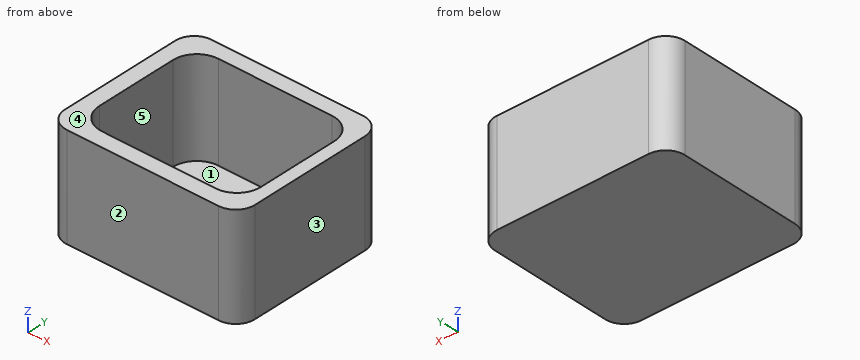
from build123d import *

# Parameters (mm, degrees)
F0_W     = 50.268072
F0_H     = 42.637728
F1_DEPTH = 27.178
F3_DEPTH = 25.4
F4_R     = 5.08
F5_R     = 5.08
F6_R     = 5.08
F7_R     = 5.08


with BuildPart() as f1:
    # F0 (on Top) → F1 (new body)
    with BuildSketch(Plane.XY):
        with Locations((-30.954471, -45.758236)):
            Rectangle(F0_W, F0_H)
    extrude(amount=F1_DEPTH)

    # F2 (on face) → F3 (cut)
    with BuildSketch(Plane.XY.offset(27.178)):
        with BuildLine():
            Line((-15.500558, -28.52626), (-45.524775, -28.52626))
            ThreePointArc((-45.524775, -28.52626), (-50.014904, -30.386132), (-51.874775, -34.87626))
            Line((-51.874775, -34.87626), (-51.874775, -56.50087))
            ThreePointArc((-51.874775, -56.50087), (-50.014904, -60.990998), (-45.524775, -62.85087))
            Line((-45.524775, -62.85087), (-15.500558, -62.85087))
            ThreePointArc((-15.500558, -62.85087), (-11.01043, -60.990998), (-9.150558, -56.50087))
            Line((-9.150558, -56.50087), (-9.150558, -34.87626))
            ThreePointArc((-9.150558, -34.87626), (-11.01043, -30.386132), (-15.500558, -28.52626))
        make_face()
    extrude(amount=-F3_DEPTH, mode=Mode.SUBTRACT)

    # F4
    f4_edges = [f1.edges().sort_by_distance(p)[0] for p in [
        (-56.088507, -67.0771, 13.589),
    ]]
    fillet(f4_edges, radius=F4_R)

    # F5
    f5_edges = [f1.edges().sort_by_distance(p)[0] for p in [
        (-5.820435, -67.0771, 13.589),
    ]]
    fillet(f5_edges, radius=F5_R)

    # F6
    f6_edges = [f1.edges().sort_by_distance(p)[0] for p in [
        (-56.088507, -24.439372, 13.589),
    ]]
    fillet(f6_edges, radius=F6_R)

    # F7
    f7_edges = [f1.edges().sort_by_distance(p)[0] for p in [
        (-5.820435, -24.439372, 13.589),
    ]]
    fillet(f7_edges, radius=F7_R)


solid = f1.part
The model under review builds one solid part; all positions refer to its coordinate system, in mm. Face numbers are marked on the shaded views. A direction names the side the tool comes from. Coordinates: 2 decimals unless noted, no trailing zeros. Loops run counter-clockwise (first coordinate to the right, second up) from the corner with the lowest first, then second, coordinate; pieces in that order, holes last. Notation, with made-up numbers: (47.25, -36.75) -> (98.25, -36.75) arc R9 ccw to (98.25, -19.75) -> close; hole circle Ø5 at (16, -21.5). An arc over 180 degrees is marked (long way). Use a Markdown table: item, result. Add a question column.
1. Add section C-C on x = -28. Write out the cut boundary in (y, z).
2. Machinability: for the marked faces 1 and 2, which of the approach directions +Z, -Z, +X, -X, +Y, -Y give a long, thin tool a straight path to every point of the face, cutting with its end or side? Answer none if there is none.
3. Add section B-B on y = -39. Write out the cut boundary in (x, z).
4. Add section A-A on z = 5.25. Write out the cut boundary in (x, y), plus the area to 3 significant figures.
5. Clearance check with flat-ended pins moving along their axes: pin 1 Ø10.5 at (x, y) = (-27.5, -46.5) entering from +Z; pin 2 Ø1.5 at (x, y) = (-23, -41) entering from -Z. State where each tip first meets the part, or that it passes through.
6. Draft analysis for pull direction X (two halves, no side actions). For the marked faces 3, 4 and 5, state which applies: pulls with the +X half, pulls with the -X half, needs draft (parallel to the pull), parting line crosses it, or undercut.
7. To check wall thickness, follow line 1 (X direction, y = -36.5, z = 23.75); line 2 (Y direction, x = -16, z = 6.5); line 3 (Z direction, x = -51, y = -54.5). State the ranges of each line that lie inside material, in increasing order.
Returned:
| question | item | result |
|---|---|---|
| 1 | outline | (-67.08, 0) -> (-24.44, 0) -> (-24.44, 27.18) -> (-28.53, 27.18) -> (-28.53, 1.78) -> (-62.85, 1.78) -> (-62.85, 27.18) -> (-67.08, 27.18) -> close |
| 2 | face 1 | +Z |
| 2 | face 2 | +Z, -Z, +X, -X, -Y |
| 3 | outline | (-56.09, 0) -> (-5.82, 0) -> (-5.82, 27.18) -> (-9.15, 27.18) -> (-9.15, 1.78) -> (-51.87, 1.78) -> (-51.87, 27.18) -> (-56.09, 27.18) -> close |
| 4 | outline | (-56.09, -62) arc R5.08 ccw to (-51.01, -67.08) -> (-10.9, -67.08) arc R5.08 ccw to (-5.82, -62) -> (-5.82, -29.52) arc R5.08 ccw to (-10.9, -24.44) -> (-51.01, -24.44) arc R5.08 ccw to (-56.09, -29.52) -> close; hole (-51.87, -56.5) arc R6.35 ccw to (-45.52, -62.85) -> (-15.5, -62.85) arc R6.35 ccw to (-9.15, -56.5) -> (-9.15, -34.88) arc R6.35 ccw to (-15.5, -28.53) -> (-45.52, -28.53) arc R6.35 ccw to (-51.87, -34.88) -> close |
| 4 | area | 689 mm² |
| 5 | pin 1 | stops at z = 1.78 |
| 5 | pin 2 | stops at z = 0 |
| 6 | face 3 | pulls with the +X half |
| 6 | face 4 | needs draft |
| 6 | face 5 | undercut |
| 7 | line 1 | x = -56.09 to -51.87, -9.15 to -5.82 |
| 7 | line 2 | y = -67.08 to -62.85, -28.53 to -24.44 |
| 7 | line 3 | z = 0 to 1.78 |
